from build123d import *

# Parameters (mm, degrees)
SKETCH1_R           = 12.7
SKETCH1_R_2         = 2.5
SKETCH1_R_3         = 1.5
BOSS_EXTRUDE1_DEPTH = 6
FILLET1_R           = 10


with BuildPart() as part:
    # Sketch1 → Boss-Extrude1 (new body)
    with BuildSketch(Plane.XY):
        Polygon((-90, 80), (90, 80), (90, -9.198698449), (0, -86.341555592), (-90, -9.198698449), align=None)
        with Locations((-70, 60)):
            Circle(SKETCH1_R, mode=Mode.SUBTRACT)
        with Locations((70, 60)):
            Circle(SKETCH1_R, mode=Mode.SUBTRACT)
        with Locations((-70, 0)):
            Circle(SKETCH1_R_2, mode=Mode.SUBTRACT)
        with Locations((70, 0)):
            Circle(SKETCH1_R_2, mode=Mode.SUBTRACT)
        with Locations((0, -60)):
            Circle(SKETCH1_R, mode=Mode.SUBTRACT)
        with Locations((-82.515790027, 47.484209973)):
            Circle(SKETCH1_R_3, mode=Mode.SUBTRACT)
        with Locations((-57.484209973, 72.515790027)):
            Circle(SKETCH1_R_3, mode=Mode.SUBTRACT)
        with Locations((-82.515790027, 12.515790027)):
            Circle(SKETCH1_R_3, mode=Mode.SUBTRACT)
        with Locations((-68.64247197, -17.647864393)):
            Circle(SKETCH1_R_3, mode=Mode.SUBTRACT)
        with Locations((-17.647864393, -61.35752803)):
            Circle(SKETCH1_R_3, mode=Mode.SUBTRACT)
        with Locations(Location((17.647864393, -61.35752803, 0), (0, 0, 180))):
            Circle(SKETCH1_R_3, mode=Mode.SUBTRACT)
        with Locations(Location((68.64247197, -17.647864393, 0), (0, 0, 180))):
            Circle(SKETCH1_R_3, mode=Mode.SUBTRACT)
        with Locations(Location((82.515790027, 12.515790027, 0), (0, 0, 180))):
            Circle(SKETCH1_R_3, mode=Mode.SUBTRACT)
        with Locations(Location((82.515790027, 47.484209973, 0), (0, 0, 180))):
            Circle(SKETCH1_R_3, mode=Mode.SUBTRACT)
        with Locations(Location((57.484209973, 72.515790027, 0), (0, 0, 180))):
            Circle(SKETCH1_R_3, mode=Mode.SUBTRACT)
    extrude(amount=BOSS_EXTRUDE1_DEPTH)

    # Fillet1
    fillet1_edges = [part.edges().sort_by_distance(p)[0] for p in [
        (90, -9.198698449, 3),
        (0, -86.341555592, 3),
        (-90, -9.198698449, 3),
    ]]
    fillet(fillet1_edges, radius=FILLET1_R)


solid = part.part
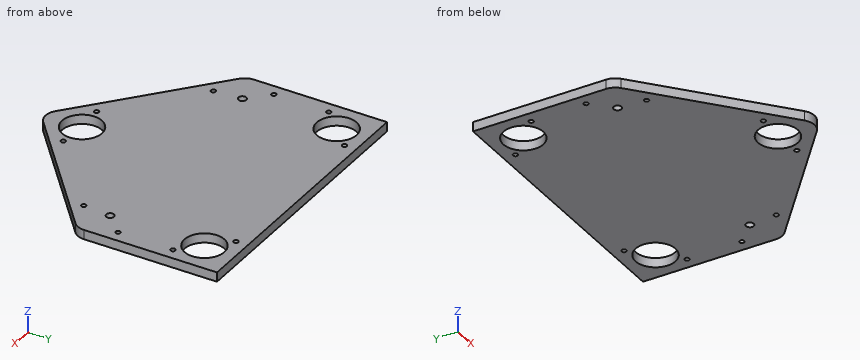
Design review of the part built by this model. Coordinates are the model's own, in mm. Give positions to 0.01 mm unless a question says otherwise; leave off trailing zeros. Order: outer loops, then holes, each group sorted by start corner. A loop starts at its lowest first (then second) coordinate and runs counter-clockwise, first axis right, second up.
1. Add section C-C, the plane y = 0. State the section outline as (x, z) points.
Solution:
outline: (-90, 0) - (-72.5, 0) - (-72.5, 6) - (-90, 6) - close; (-67.5, 0) - (67.5, 0) - (67.5, 6) - (-67.5, 6) - close; (72.5, 0) - (90, 0) - (90, 6) - (72.5, 6) - close
2. Add section D-D, the plane z = 2.25. State how many separate pieces and enclosed holes the cut face has, then the cut area to 3 significant figures.
Solution:
separate pieces: 1
enclosed holes: 15
area: 21,300 mm2
3. For pin 1 Ø2 at (x, z) = (-5, 4.5) entering from -Y; pin 2 Ø1.5 at (y, z) = (-25, 4) entering from +X; pin 3 Ø1.5 at (x, z) = (-6.5, 2) entering from -Y; pin 4 Ø5 at (x, y) = (-68.64, -17.65) entering from +Z, all flat-tipped, find the tip position at first contact; note any pin that passes through.
Solution:
pin 1: stops at y = -82.34
pin 2: stops at x = 72.44
pin 3: stops at y = -81.35
pin 4: stops at z = 6
4. Add section A-A, the plane y = 60. State the section outline as (x, z) points, then the cut area to 3 significant figures.
Solution:
outline: (-90, 0) - (-82.7, 0) - (-82.7, 6) - (-90, 6) - close; (-57.3, 0) - (57.3, 0) - (57.3, 6) - (-57.3, 6) - close; (82.7, 0) - (90, 0) - (90, 6) - (82.7, 6) - close
area: 775 mm2
5. To check wall thickness, follow L1, parallel to X at y = 13, z = 4.2; L2, parallel to X at y = -16.5, z = 5; L3, parallel to X at y = -64.5, z = 5.1. State the ranges of each line that lie inside material, in increasing order.
Solution:
L1: x = -90 to -83.94, -81.1 to 81.1, 83.94 to 90
L2: x = -81.48 to -69.61, -67.68 to 67.68, 69.61 to 81.48
L3: x = -25.48 to -11.88, 11.88 to 25.48
6. Add section B-B, the plane x = 0. State the section outline as (y, z) points.
Solution:
outline: (-83.17, 0) - (-72.7, 0) - (-72.7, 6) - (-83.17, 6) - close; (-47.3, 0) - (80, 0) - (80, 6) - (-47.3, 6) - close
